```python
from build123d import *

# Parameters (mm, degrees)
F1_DEPTH       = 25
F3_D           = 13.2
F3_CBORE_D     = 19.25
F3_CBORE_DEPTH = 0
F5_D           = 13.2
F5_CBORE_D     = 19.25
F5_CBORE_DEPTH = 0
F6_W           = 40
F6_H           = 30.5
F7_DEPTH       = 30
F8_R           = 16
F9_DEPTH       = 30
F10_R          = 16
F11_DEPTH      = 30


with BuildPart() as f1:
    # F0 (on Front) → F1 (new body, symmetric)
    with BuildSketch(Plane.XZ):
        with BuildLine():
            Line((25, -25.5), (25, -40))
            Line((25, -40), (10.5, -40))
            ThreePointArc((10.5, -40), (25, -54.5), (39.5, -40))
            ThreePointArc((39.5, -40), (35.2530483272, -29.7469516728), (25, -25.5))
        make_face()
        with BuildLine():
            Line((10.5, -40), (25, -40))
            Line((25, -40), (25, -25.5))
            ThreePointArc((25, -25.5), (14.7469516728, -29.7469516728), (10.5, -40))
        make_face()
        with BuildLine():
            Line((-25, -40), (10.5, -40))
            ThreePointArc((10.5, -40), (14.7469516728, -29.7469516728), (25, -25.5))
            Line((25, -25.5), (25, 25.5))
            ThreePointArc((25, 25.5), (14.7469516728, 29.7469516728), (10.5, 40))
            Line((10.5, 40), (-25, 40))
            Line((-25, 40), (-25, 14.2162181315))
            ThreePointArc((-25, 14.2162181315), (-14.9640357801, 9.8540823977), (-10.8347666082, -0.279916916))
            ThreePointArc((-10.8347666082, -0.279916916), (-14.9640357801, -10.4139162298), (-25, -14.7760519636))
            Line((-25, -14.7760519636), (-25, -40))
        make_face()
        with BuildLine():
            ThreePointArc((10.5, 40), (14.7469516728, 29.7469516728), (25, 25.5))
            Line((25, 25.5), (25, 40))
            Line((25, 40), (10.5, 40))
        make_face()
        with BuildLine():
            Line((25, 40), (25, 25.5))
            ThreePointArc((25, 25.5), (35.2530483272, 29.7469516728), (39.5, 40))
            ThreePointArc((39.5, 40), (25, 54.5), (10.5, 40))
            Line((10.5, 40), (25, 40))
        make_face()
        with BuildLine():
            ThreePointArc((-25, 14.2162181315), (-39.8347666082, -0.279916916), (-25, -14.7760519636))
            Line((-25, -14.7760519636), (-25, 14.2162181315))
        make_face()
        with BuildLine():
            Line((-25, 14.2162181315), (-25, -14.7760519636))
            ThreePointArc((-25, -14.7760519636), (-14.9640357801, -10.4139162298), (-10.8347666082, -0.279916916))
            ThreePointArc((-10.8347666082, -0.279916916), (-14.9640357801, 9.8540823977), (-25, 14.2162181315))
        make_face()
    extrude(amount=F1_DEPTH, both=True)

    # F3 (through all)
    with Locations(Plane.XZ.offset(25)):
        with Locations((25, 40), (-25.3347666082, -0.279916916), (25, -40)):
            CounterBoreHole(F3_D / 2, F3_CBORE_D / 2, F3_CBORE_DEPTH)

    # F5 (through all)
    with Locations(Plane.XY.offset(40)):
        with Locations((-13, 9.3407420599), (5.0832007976, -9.3407420599)):
            CounterBoreHole(F5_D / 2, F5_CBORE_D / 2, F5_CBORE_DEPTH)

    # F6 (on face) → F7 (cut)
    with BuildSketch(Plane.XZ.offset(25)):
        with Locations((9.9, 0)):
            Rectangle(F6_W, F6_H)
    extrude(amount=-F7_DEPTH, mode=Mode.SUBTRACT)

    # F8 (on face) → F9 (cut)
    with BuildSketch(Plane.XY.offset(-15.25)):
        with Locations((5.0832007976, -9.3407420599)):
            Circle(F8_R)
    extrude(amount=F9_DEPTH, mode=Mode.SUBTRACT)

    # F10 (on face) → F11 (cut)
    with BuildSketch(Plane.XZ.offset(25)):
        with Locations((25, 40)):
            Circle(F10_R)
        with Locations((25, -40)):
            Circle(F10_R)
    extrude(amount=-F11_DEPTH, mode=Mode.SUBTRACT)


solid = f1.part
```
Here's how the part is built. I have some questions about the finished solid (model axes, mm). A direction names the side the tool comes from. Coordinates: 2 decimals unless noted, no trailing zeros. Order: outer loops, then holes, each group sorted by start corner. A loop starts at its lowest first (then second) coordinate and runs counter-clockwise, first axis right, second up. Notation, with made-up numbers: (-22, -4.75) - (34, -4.75) arc R13 cw to (34, 13.25) - close; hole circle Ø2 at (53, -12.75). An arc over 180 degrees is marked (long way). One line per question, with ' | ' between items.
(1) Suppose I cut it at B-B on z = -32. List the corners of the cut face in (x, y) for me.
Report:
outline: (-25, -25) - (11.14, -25) - (11.14, -11.95) arc R6.6 cw (long way) to (11.14, -6.73) - (11.14, 5) - (37.09, 5) - (37.09, 25) - (-25, 25) - close; hole circle Ø13.2 at (-13, 9.34)
(2) For faces 1 (the cylindrical face through (-10.917, -9.269, -0.46)), 2 (the flat face through (-25, 0, 27)), 3 (the cylindrical face through (13.811, -10.21, -28.563)), 4 (the flat face through (16, 5, 0)), which set-ups out of +Z, -Z, +X, -X, +Y, -Y let a thin tool reach every point of the face, with its end or its side?
Report:
face 1: +X | face 2: +Z, -X, +Y, -Y | face 3: -Z, +X, -Y | face 4: +X, -Y
(3) Will these pins go through, and if not, where does the flat tip stop? pin 1 (15 mm diameter, centred on x = -13, y = 9.34, fed in from +Z); pin 2 (24.5 mm diameter, centred on x = 23.5, z = -33, fed in from -Y); pin 3 (20 mm diameter, centred on y = -0.5, z = -29, fed in from -X); pin 4 (4 mm diameter, centred on x = -31.5, y = 11, fed in from -Z).
Report:
pin 1: stops at z = 40 | pin 2: stops at y = -25 | pin 3: stops at x = -25 | pin 4: stops at z = -14.17
(4) Suppose I cut it at C-C on x = 20. List the corners of the cut face in (y, z) for me, and give its area (3 significant figures).
Report:
outline: (-25, -24.8) - (5, -24.8) - (5, -35.69) - (25, -35.69) - (25, 35.69) - (5, 35.69) - (5, 24.8) - (-25, 24.8) - (-25, 15.25) - (5, 15.25) - (5, -15.25) - (-25, -15.25) - close; (5, -53.61) - (25, -53.61) - (25, -44.31) - (5, -44.31) - close; (5, 44.31) - (25, 44.31) - (25, 53.61) - (5, 53.61) - close | area: 2,370 mm2
(5) Suppose I cut it at A-A on x = -13. List the corners of the cut face in (y, z) for me.
Report:
outline: (-25, -40) - (2.74, -40) - (2.74, 40) - (-25, 40) - close; (15.94, -40) - (25, -40) - (25, 40) - (15.94, 40) - close
(6) If I drill on L1, parallel to Y at x = -13, z = 12; L2, parallel to X at y = 15, z = 36; L3, parallel to X at y = 5.5, z = -36.5, over which ranges is the centre line in solid material (lowest first)?
Report:
L1: y = -25 to 2.74, 15.94 to 25 | L2: x = -25 to -16.4, -9.6 to 19.75, 30.25 to 38.94 | L3: x = -25 to -18.37, -7.63 to 19.4, 30.6 to 39.07
(7) Suppose I cut it at D-D on x = 29. List the corners of the cut face in (y, z) for me.
Report:
outline: (5, -53.94) - (25, -53.94) - (25, -45.25) - (5, -45.25) - close; (5, -34.75) - (25, -34.75) - (25, -26.06) - (5, -26.06) - close; (5, 26.06) - (25, 26.06) - (25, 34.75) - (5, 34.75) - close; (5, 45.25) - (25, 45.25) - (25, 53.94) - (5, 53.94) - close
(8) If we mould it in two halves opening along Y, with no side actions, what happens to faces 5 (the flat face through (-1, 25, 1)), 6 (the flat face through (-25, 0, -27)), 7 (the cylindrical face through (-6.406, 9.631, -0.56)), 8 (the cylindrical face through (-1.212, -7.358, 27.452))? For each: pulls with the +Y half, pulls with the -Y half, needs draft (parallel to the pull), parting line crosses it, or undercut.
Report:
face 5: pulls with the +Y half | face 6: needs draft | face 7: undercut | face 8: undercut
